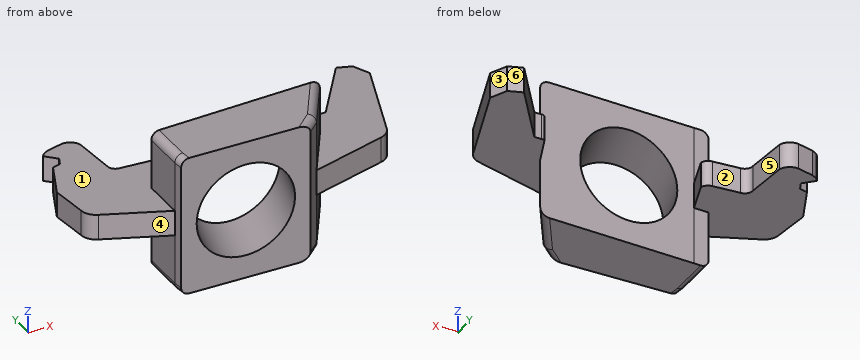
Autodesk Fusion 360 part; units mm, degrees
sketch "Sketch1" plane through (0, 0, 0) normal (0, 0, 1) x (1, 0, 0)
  line L0 (-26.67, 1.27) -> (-24.1476, 7.2462)
  line L1 (-24.1476, 7.2462) -> (-22.86, 7.62)
  line L2 (-22.86, 7.62) -> (-22.315, 8.9113)
  line L3 (-22.315, 8.9113) -> (-24.003, 10.541)
  line L4 (-23.5873, 11.0942) -> (-22.733, 11.557)
  line L5 (-22.733, 11.557) -> (-20.2207, 12.194)
  arc A0 (-17.9561, 10.8132) -> (-20.2207, 12.194) centre (-19.9, 10.1725) ccw
  arc A1 (-17.272, 4.064) -> (-16.002, 2.794) centre (-16.002, 4.064) ccw
  arc A2 (-10.414, 1.524) -> (-11.684, 2.54) centre (-11.7021, 1.2156) ccw
  line L6 (-16.002, 2.794) -> (-11.684, 2.54)
  line L7 (-17.9561, 10.8132) -> (-17.272, 4.064)
  line L8 (-10.414, 1.524) -> (-12.0756, -3.7274)
  line L9 (-12.0756, -3.7274) -> (12.8223, -2.4887)
  line L10 (12.8223, -2.4887) -> (14.564, 2.0647)
  arc A3 (15.1915, 2.428) -> (14.564, 2.0647) centre (15.0967, 1.8682) ccw
  line L11 (15.1915, 2.428) -> (16.3321, 2.428)
  line L12 (16.3321, 2.428) -> (23.0225, 12.1287)
  line L13 (23.0225, 12.1287) -> (25.292, 11.3722)
  line L14 (25.292, 11.3722) -> (26.5825, 8.7022)
  line L15 (26.5825, 8.7022) -> (21.9101, -5.3151)
  arc A4 (20.1504, -6.9936) -> (21.9101, -5.3151) centre (19.4463, -4.4938) ccw
  arc A5 (-25.9136, -4.4938) -> (-24.2756, -6.6881) centre (-23.4373, -4.3537) ccw
  line L16 (-26.67, 1.27) -> (-25.9136, -4.4938)
  line L17 (-24.2756, -6.6881) -> (-14.3296, -10.6903)
  line L18 (-14.3296, -10.6903) -> (-14.1291, -12.218)
  line L19 (-14.1291, -12.218) -> (6.2698, -12.218)
  line L20 (6.2698, -12.218) -> (8.1283, -10.465)
  line L21 (8.1283, -10.465) -> (20.1504, -6.9936)
  line L22 (-12.0756, -3.7274) -> (-14.4554, -3.8458)
  line L23 (-14.4554, -3.8458) -> (-14.3296, -10.6903)
  line L24 (12.8223, -2.4887) -> (8.1283, -10.465)
  line L25 (-24.003, 10.541) -> (-23.5873, 11.0942)
extrude "Extrude1" add sketch "Sketch1" along normal mid plane 4.064 contours L0 L1 L2 L3 L4 L5 A0 A1 A2 L6 L7 L8 A5 L16 L17 L22 L23 L25 | L10 A3 L11 L12 L13 L14 L15 A4 L21 L24 makes body 1 at (-19.0192, -1.7813, 2.032) makes body 2 at (21.6083, 1.9384, 2.032)
extrude "Extrude2" add sketch "Sketch1" along normal mid plane 22.352 contours L9 L18 L19 L20 L22 L23 L24 bodies 1 2
ref_plane "WorkPlane1" through (6.2698, -12.218, 0) normal (0.2588, 0.9659, 0) x (0, 0, 1)
sketch "Sketch4" plane through (6.2698, -12.218, 0) normal (0.2588, 0.9659, 0) x (0, 0, 1)
  line L0 (-11.176, -19.7038) -> (11.176, -19.7038)
  line L1 (-11.176, 0) -> (-11.176, -19.7038) construction
  circle A0 centre (0, -9.8486) radius 7.493
  point P0 (-11.176, 0)
  point P1 (-11.176, 0)
  point P2 (11.176, 0)
  point P3 (0, -9.8486)
  dimension "d6" = 22.352
  dimension "d7" = 19.7038
  dimension "d8" = 9.8552
  dimension "d9" = 11.176
  dimension "d10" = 14.986
extrude "Extrude3" cut sketch "Sketch4" along normal through all and the other way through all bodies 1
fillet "Fillet1" radius 1.27 8 edges at (10.4753, -6.4768, 11.176) (7.1991, -11.3415, 11.176) (-14.3925, -7.268, 11.176) (-14.2293, -11.4541, 11.176) (-14.3925, -7.268, -11.176) (-14.2293, -11.4541, -11.176) (10.4753, -6.4768, -11.176) (7.1991, -11.3415, -11.176) on bodies 1
Geometry: final body of the model. Coordinates: model frame, mm. Face numbers are marked on the shaded views. A direction names the side the tool comes from. Coordinates: 2 decimals unless noted, no trailing zeros. Order: outer loops, then holes, each group sorted by start corner. A loop starts at its lowest first (then second) coordinate and runs counter-clockwise, first axis right, second up.
(1) Material intervals for probe 1 along Z at (x, y) = (17.5, 2.75); probe 2 along X at (y, z) = (3.5, -2); probe 3 along X at (y, z) = (5.5, 1), sorted ascending.
(2) Section query B-B (z = 8.75). Return the cut outline in (x, y) (3 decimals).
(3) First-contact query: pin 1 (4 mm diameter, centred on x = 20.5, y = -5.5, fed in from +Z); pin 2 (8 mm diameter, centred on y = -2.5, z = 7, fed in from +X); pin 3 (10 mm diameter, centred on y = -4.5, z = -2, fed in from -X); pin 4 (5 mm diameter, centred on x = 16.5, z = -5.5, fed in from -Y). Flat tips, straight axial feed; report the tip coordinate or a pass-through.
(4) Section query D-D (z = 3). Return the cut outline in (x, y) (3 decimals).
(5) Draft query along X for the marked faces 1, 2, 3 and 4. Return one class per face: pulls with the +X half, pulls with the -X half, needs draft (parallel to the pull), parting line crosses it, or undercut.
(6) Section query C-C (y = 4.75). Return the cut outline in (x, z).
(7) Access query for the marked faces 5 and 6. Directions: +Z, -Z, +X, -X, +Y, -Y. A direction counts if a zero-diameter tool reaches every point of the face in a straight line with its end or side. Return the directions, or none.
Solution:
1. probe 1: z = -2.03 to 2.03
1. probe 2: x = -25.73 to -17.14, 17.07 to 24.85
1. probe 3: x = -24.88 to -17.42, 18.45 to 25.52
2. outline: (-14.455, -3.846) - (-14.33, -10.69) - (-14.129, -12.218) - (6.27, -12.218) - (8.128, -10.465) - (12.822, -2.489) - (-12.076, -3.727) - close
3. pin 1: stops at z = 2.03
3. pin 2: stops at x = 12.82
3. pin 3: stops at x = -26.57
3. pin 4: passes through
4. outline: (-14.455, -3.846) - (-14.33, -10.69) - (-14.129, -12.218) - (-11.035, -12.218) - (-8.715, -3.56) - (-12.076, -3.727) - close; (3.182, -12.218) - (6.27, -12.218) - (8.128, -10.465) - (12.822, -2.489) - (5.694, -2.843) - close
5. face 1: needs draft
5. face 2: undercut
5. face 3: pulls with the +X half
5. face 4: pulls with the -X half
6. outline: (-25.2, -2.03) - (-17.34, -2.03) - (-17.34, 2.03) - (-25.2, 2.03) - close; (17.93, -2.03) - (25.27, -2.03) - (25.27, 2.03) - (17.93, 2.03) - close
7. face 5: +Z, -Z, +Y
7. face 6: +Z, -Z, +X, +Y
